Geometry: final body of the model. Coordinates: model frame, mm. Give positions to 0.01 mm unless a question says otherwise; leave off trailing zeros. Order: outer loops, then holes, each group sorted by start corner. A loop starts at its lowest first (then second) coordinate and runs counter-clockwise, first axis right, second up. Notation, with made-up numbers: (89, 85) -> (101, 85) arc R21 cw to (101, 114) -> close; hole circle Ø10 at (21.5, -21.5). An arc over 180 degrees is marked (long way). One line per question, with ' | ' between items.
from build123d import *

# Parameters (mm, degrees)
SKETCH1_R           = 1.65
BOSS_EXTRUDE1_DEPTH = 3
SKETCH2_R           = 1.6
BOSS_EXTRUDE2_DEPTH = 3
SKETCH3_R           = 0.95
CUT_EXTRUDE1_DEPTH  = 99.001298809


with BuildPart() as part:
    # Sketch1 → Boss-Extrude1 (new body)
    with BuildSketch(Plane(origin=(0, 0, 0), x_dir=(1, 0, 0), z_dir=(0, 1, 0))):
        with BuildLine():
            ThreePointArc((-4.721587007, -63.38854654), (0, -75.556390977), (4.721587007, -63.38854654))
            ThreePointArc((4.721587007, -63.38854654), (2.011300437, -57.650074902), (4.111268391, -51.661264952))
            ThreePointArc((4.111268391, -51.661264952), (4.746967497, -50.785668514), (5.198942096, -49.802560464))
            ThreePointArc((5.198942096, -49.802560464), (4.579991672, -48.53098649), (3.308417698, -49.149936914))
            ThreePointArc((3.308417698, -49.149936914), (0, -51.507845701), (-3.308417698, -49.149936914))
            ThreePointArc((-3.308417698, -49.149936914), (-4.579991672, -48.53098649), (-5.198942096, -49.802560464))
            ThreePointArc((-5.198942096, -49.802560464), (-4.746967497, -50.785668514), (-4.111268391, -51.661264952))
            ThreePointArc((-4.111268391, -51.661264952), (-2.011300437, -57.650074902), (-4.721587007, -63.38854654))
        make_face()
        with Locations(Location((0, -68.556390977, 0), (0, 0, 270))):
            Circle(SKETCH1_R, mode=Mode.SUBTRACT)
    extrude(amount=BOSS_EXTRUDE1_DEPTH)

    # Sketch2 → Boss-Extrude2 (add)
    with BuildSketch(Plane.XZ):
        with BuildLine():
            ThreePointArc((-4.029144211, 90.885477552), (0, 97.704936254), (4.029144211, 90.885477552))
            ThreePointArc((4.029144211, 90.885477552), (2.054398705, 81.663604808), (5.501134896, 72.885076096))
            ThreePointArc((5.501134896, 72.885076096), (0, 75.556390977), (-5.501134896, 72.885076096))
            ThreePointArc((-5.501134896, 72.885076096), (-2.054398705, 81.663604808), (-4.029144211, 90.885477552))
        make_face()
        with Locations(Location((0, 93.104936254, 0), (0, 0, 270))):
            Circle(SKETCH2_R, mode=Mode.SUBTRACT)
    extrude(amount=-BOSS_EXTRUDE2_DEPTH)

    # Sketch3 → Cut-Extrude1 (cut, through all)
    with BuildSketch(Plane(origin=(0, 3, 0), x_dir=(1, 0, 0), z_dir=(0, 1, 0))):
        with Locations(Location((0, -65.506390977, 0), (0, 0, 270))):
            Circle(SKETCH3_R)
        with Locations(Location((2.641377482, -67.031390977, 0), (0, 0, 270))):
            Circle(SKETCH3_R)
        with Locations(Location((2.641377482, -70.081390977, 0), (0, 0, 270))):
            Circle(SKETCH3_R)
        with Locations(Location((0, -71.606390977, 0), (0, 0, 270))):
            Circle(SKETCH3_R)
        with Locations(Location((-2.641377482, -70.081390977, 0), (0, 0, 270))):
            Circle(SKETCH3_R)
        with Locations(Location((-2.641377482, -67.031390977, 0), (0, 0, 270))):
            Circle(SKETCH3_R)
    extrude(amount=-CUT_EXTRUDE1_DEPTH, mode=Mode.SUBTRACT)


solid = part.part
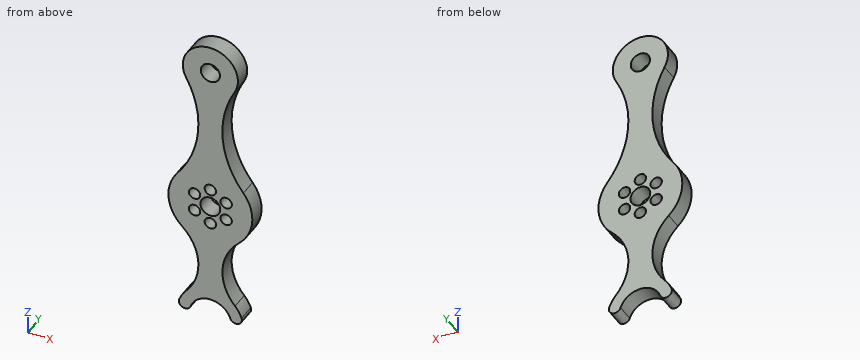
1) Section B-B on z = 65. Return loops of the section in (x, y).
Check result:
outline: (-6.03, 0) -> (-0.8, 0) -> (-0.8, 3) -> (-6.03, 3) -> close; (0.8, 0) -> (6.03, 0) -> (6.03, 3) -> (0.8, 3) -> close
2) Contact query for flat-ended pins moving along their axis: pin 1 Ø1.5 at (y, z) = (2, 91) entering from -X; pin 2 Ø1.1 at (x, z) = (0, 71.61) entering from +Y; pin 3 Ø1 at (x, y) = (-2.5, 2) entering from +Z. Output: stop coordinate, or through.
Check result:
pin 1: stops at x = -4.4 | pin 2: passes through | pin 3: stops at z = 97.25
3) Section D-D on z = 56.5. Return loops of the section in (x, y), plus the area to 3 significant figures.
Check result:
outline: (-2.03, 0) -> (2.03, 0) -> (2.03, 3) -> (-2.03, 3) -> close | area: 12.2 mm^2
4) Section C-C on y = 1.8. Count the separate pieces of the cut face and the enclosed holes in it, plus the area to 3 significant figures.
Check result:
separate pieces: 1 | enclosed holes: 8 | area: 325 mm^2
5) Material intervals for probe 1 along Z at (x, y) = (-4, 0.25); probe 2 along Z at (x, y) = (-0.5, 1.1); probe 3 along X at (y, z) = (1.05, 93), sorted ascending. Write a range as from..to.
Check result:
probe 1: z = 48.51..51.79, 62.64..75.16, 90.83..95.38 | probe 2: z = 51.47..64.7, 66.31..66.98, 70.13..70.8, 72.41..91.59, 94.62..97.68 | probe 3: x = -4.6..-1.6, 1.6..4.6
6) Section A-A on x = 0. Return loops of the section in (y, z).
Check result:
outline: (0, 51.51) -> (3, 51.51) -> (3, 64.56) -> (0, 64.56) -> close; (0, 66.46) -> (3, 66.46) -> (3, 66.91) -> (0, 66.91) -> close; (0, 70.21) -> (3, 70.21) -> (3, 70.66) -> (0, 70.66) -> close; (0, 72.56) -> (3, 72.56) -> (3, 91.5) -> (0, 91.5) -> close; (0, 94.7) -> (3, 94.7) -> (3, 97.7) -> (0, 97.7) -> close
